from build123d import *

# Parameters (mm, degrees)
ESQUISSE1_W             = 200
ESQUISSE1_H             = 75
BOSS_EXTRU_1_DEPTH      = 10
CONG_1_R                = 10
ESQUISSE2_W             = 20
ESQUISSE2_H             = 40
ENL_V_MAT_EXTRU_1_DEPTH = 10
ESQUISSE3_W             = 20
ESQUISSE3_H             = 10
ENL_V_MAT_EXTRU_2_DEPTH = 1
D_GAGEMENT_M21_D        = 2.4


with BuildPart() as part:
    # Esquisse1 → Boss.-Extru.1 (new body)
    with BuildSketch(Plane(origin=(0, 0, 0), x_dir=(1, 0, 0), z_dir=(0, 1, 0))):
        with Locations((100, 37.5)):
            Rectangle(ESQUISSE1_W, ESQUISSE1_H)
    extrude(amount=BOSS_EXTRU_1_DEPTH)

    # Cong_1
    cong_1_edges = [part.edges().sort_by_distance(p)[0] for p in [
        (0, 5, -75),
        (200, 5, -75),
        (200, 5, 0),
        (0, 5, 0),
    ]]
    fillet(cong_1_edges, radius=CONG_1_R)

    # Esquisse2 → Enl_v. mat.-Extru.1 (cut)
    with BuildSketch(Plane(origin=(0, 10, 0), x_dir=(1, 0, 0), z_dir=(0, 1, 0))):
        with Locations((25, 52.5)):
            Rectangle(ESQUISSE2_W, ESQUISSE2_H)
        with Locations((175, 52.5)):
            Rectangle(ESQUISSE2_W, ESQUISSE2_H)
    extrude(amount=-ENL_V_MAT_EXTRU_1_DEPTH, mode=Mode.SUBTRACT)

    # Esquisse3 → Enl_v. mat.-Extru.2 (cut)
    with BuildSketch(Plane.XZ):
        with Locations((100, -10)):
            Rectangle(ESQUISSE3_W, ESQUISSE3_H)
    extrude(amount=-ENL_V_MAT_EXTRU_2_DEPTH, mode=Mode.SUBTRACT)

    # D_gagement M21 (through all)
    with Locations(Plane(origin=(0, 1, 0), x_dir=(-1, 0, 0), z_dir=(0, -1, 0))):
        with Locations((-106, 10), (-94, 10)):
            Hole(D_GAGEMENT_M21_D / 2)


solid = part.part
Geometry check sheet. Reference: the model listing, model coordinates, mm. A direction names the side the tool comes from. Give positions to 0.01 mm unless a question says otherwise; leave off trailing zeros. Order: outer loops, then holes, each group sorted by start corner. A loop starts at its lowest first (then second) coordinate and runs counter-clockwise, first axis right, second up.
1) Tool access check on faces 1 (the flat face through (175, 5, -32.5)), 2 (the flat face through (100, 1, -10)), 3 (the flat face through (99, 5, -75)). Record the directions out of +Z, -Z, +X, -X, +Y, -Y that give a thin tool (end or side, any length) a straight path to the whole face; none if there is none.
Results are:
face 1: +Y, -Y
face 2: -Y
face 3: -Z, +X, -X, +Y, -Y
2) Draft check along X on faces 4 (the flat face through (99, 5, 0)), 5 (the cylindrical face through (2.85, 5.07, -71.99)), 6 (the flat face through (175, 5, -72.5)), 7 (the flat face through (200, 5, -37)). Enter one of: released by +X, released by -X, zero draft, split by the parting line, or undercut.
Results are:
face 4: zero draft
face 5: released by -X
face 6: undercut
face 7: released by +X
3) Cross-section at B-B (y = 8). Record the boundary of the cut face in (x, z).
Results are:
outline: (0, -65) arc R10 ccw to (10, -75) - (190, -75) arc R10 ccw to (200, -65) - (200, -10) arc R10 ccw to (190, 0) - (10, 0) arc R10 ccw to (0, -10) - close; hole (15, -72.5) - (35, -72.5) - (35, -32.5) - (15, -32.5) - close; hole circle Ø2.4 at (94, -10); hole circle Ø2.4 at (106, -10); hole (165, -72.5) - (185, -72.5) - (185, -32.5) - (165, -32.5) - close
4) Material ranges on probe 1 along X at (y, z) = (4.5, -56); probe 2 along Z at (x, y) = (106, 6.5); probe 3 along Z at (x, y) = (17, 3), recorded low to high.
Results are:
probe 1: x = 0 to 15, 35 to 165, 185 to 200
probe 2: z = -75 to -11.2, -8.8 to 0
probe 3: z = -75 to -72.5, -32.5 to 0
5) Cross-section at A-A (z = -38). Record the boundary of the cut face in (x, y), then the cut area to 3 significant figures.
Results are:
outline: (0, 0) - (15, 0) - (15, 10) - (0, 10) - close; (35, 0) - (165, 0) - (165, 10) - (35, 10) - close; (185, 0) - (200, 0) - (200, 10) - (185, 10) - close
area: 1,600 mm2
